Part print with two shaded views. Sizes in mm from the minimum x, y, z corner. A direction names the side the tool comes from. Give positions to 0.01 mm unless a question says otherwise; leave off trailing zeros. Loops run counter-clockwise (first coordinate to the right, second up) from the corner with the lowest first, then second, coordinate; pieces in that order, holes last. Notation, with made-up numbers: (-27.75, -7) -> (-22.75, -7) arc R30 ccw to (-22.75, 22) -> close; hole circle Ø11 at (9.5, 76.5). An arc over 180 degrees is marked (long way). One line per question, with ' | ' between items. Start each with the question number.
(1) Flat gauge pins, fed straight in: pin 1 Ø6 at (y, z) = (16.5, 8) entering from +X; pin 2 Ø6 at (x, z) = (13.5, 21.5) entering from +Y; pin 3 Ø6 at (x, z) = (64, 31) entering from -Y. Where does each tip first touch, or does it go through?
(2) 3-axis set-ups, long thin cutter, end or side, ignore diameter. For the marked faces 1, 2 and 3: which of +Z, -Z, +X, -X, +Y, -Y reach the whole face in a straight line?
(3) Slice it at B-B, the plane x = 20. Write the cut outline in (y, z).
(4) Slice it at A-A, the plane z = 20. Write the cut outline in (x, y), then the cut area to 3 significant figures.
(5) Slice it at D-D, the plane y = 14. Write the cut outline in (x, z), then the cut area to 3 significant figures.
(6) Drill centre lines: L1, parallel to Z at x = 68, y = 52.2; L2, parallel to Y at x = 15.5, z = 2.5; L3, parallel to X at y = 24.5, z = 8.5. Where is each one in solid material? Low to high. Write a range as from..to.
(7) Slice it at C-C, the plane z = 28. Write the cut outline in (x, y).
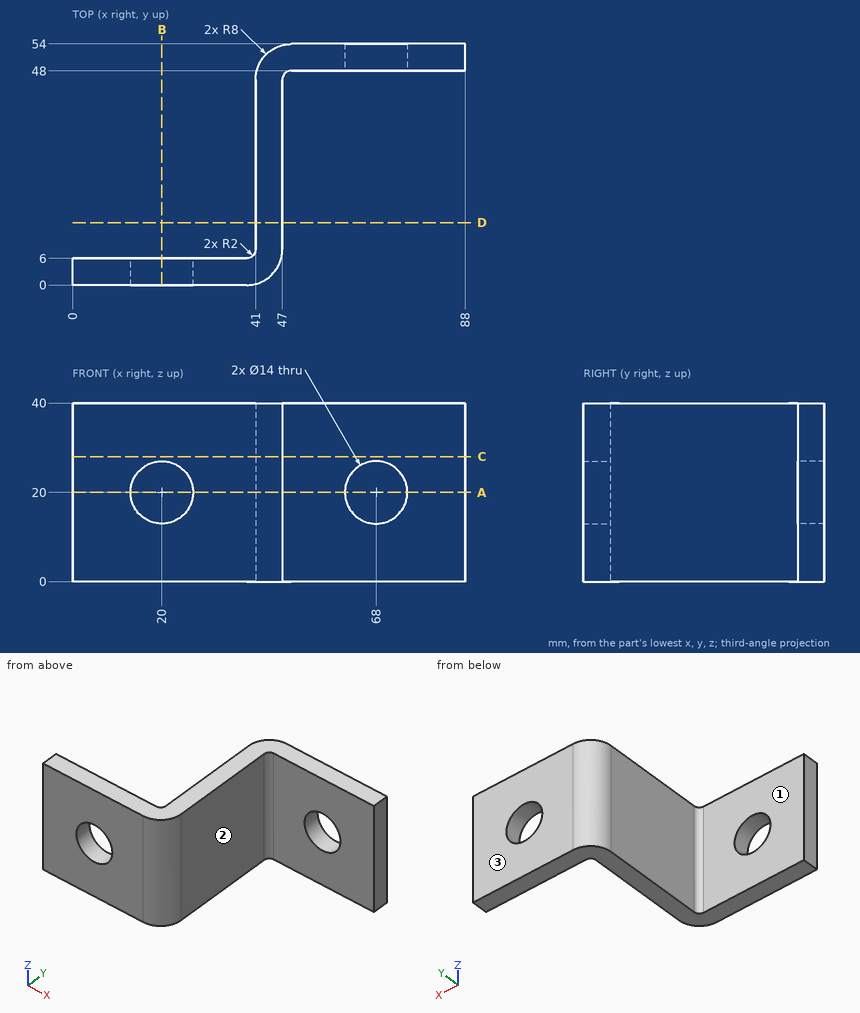
Final values:
1) pin 1: x = 47 | pin 2: y = 6 | pin 3: y = 48
2) face 1: +Z, -Z, -X, +Y | face 2: +Z, -Z, +X, -Y | face 3: +Z, -Z, +X, -X, +Y
3) outline: (0, 0) -> (6, 0) -> (6, 13) -> (0, 13) -> close; (0, 27) -> (6, 27) -> (6, 40) -> (0, 40) -> close
4) outline: (0, 0) -> (13, 0) -> (13, 6) -> (0, 6) -> close; (27, 0) -> (39, 0) arc R8 ccw to (47, 8) -> (47, 46) arc R2 cw to (49, 48) -> (61, 48) -> (61, 54) -> (49, 54) arc R8 ccw to (41, 46) -> (41, 8) arc R2 cw to (39, 6) -> (27, 6) -> close; (75, 48) -> (88, 48) -> (88, 54) -> (75, 54) -> close | area: 622 mm2
5) outline: (41, 0) -> (47, 0) -> (47, 40) -> (41, 40) -> close | area: 240 mm2
6) L1: 0..13, 27..40 | L2: 0..6 | L3: 41..47
7) outline: (0, 0) -> (39, 0) arc R8 ccw to (47, 8) -> (47, 46) arc R2 cw to (49, 48) -> (88, 48) -> (88, 54) -> (49, 54) arc R8 ccw to (41, 46) -> (41, 8) arc R2 cw to (39, 6) -> (0, 6) -> close
